The model under review builds one solid part; all positions refer to its coordinate system, in mm. A direction names the side the tool comes from. Round coordinates to 2 decimals unless told otherwise and drop trailing zeros. Order: outer loops, then holes, each group sorted by start corner. A loop starts at its lowest first (then second) coordinate and runs counter-clockwise, first axis right, second up. Notation, with made-up numbers: M 0.5,38.25 L 6.5,38.25 A16 ccw 6.5,62.25 Z; hole C 52,41.5 d8. An arc over 180 degrees is marked long. Use a Markdown table: item, result. Add a question column.
1. The part is to be moulded in two halves that separate along Y. For faces 1 (the cylindrical face through (43.544, 9.789, 10.874)), 2 (the cylindrical face through (-42.526, -11.023, -1.496)), 3 (the flat face through (44, 6.215, 16)), 4 (the flat face through (-41.952, -7, 10)), say which applies: +Y half, -Y half, draft (parallel to the pull), parting line (faces both ways), or undercut.
2. Consider section D-D on y = -10. State the section outline as (x, z) points, then the cut area to 3 significant figures.
3. Insertion check: P1, Ø0.6, axis at x = 44, y = 0.5, coming from the +Z side; P2, Ø0.6, axis at x = 44, z = 17, coming from the +Y side; P3, Ø2, axis at x = -43.5, z = 15, coming from the +Y side. Each pin has a flat end and moves straight along its axis. Give the tip position at first contact, or say it passes through.
4. Consider section C-C on x = 15.5. State the section outline as (y, z) points.
5. For faces 5 (the flat face through (44, 1, 10)), 6 (the flat face through (0, -11, 0)), 7 (the flat face through (-43, -17.785, 16)), list the 3-axis set-ups (+Z, -Z, +X, -X, +Y, -Y) from which the entire face can be reached by the end or side of a thin tool; tool diameter is ignored.
6. To check wall thickness, follow probe 1 along Y at (x, z) = (-22, 3.5); probe 2 along X at (y, z) = (-15, 11.5); probe 3 along Z at (x, y) = (4, -22). State the ranges of each line that lie inside material, in increasing order.
7. Consider section A-A on z = 15. State the section outline as (x, y) points.
8. Consider section B-B on z = 4.25. State the section outline as (x, y) points.
from build123d import *

# Parameters (mm, degrees)
F0_W      = 89
F0_H      = 44
F0_W_2    = 85
F0_H_2    = 40
F1_DEPTH  = 20
F2_W      = 89
F2_H      = 44
F2_W_2    = 85
F2_H_2    = 40
F3_DEPTH  = 3
F4_R      = 5
F5_R      = 3
F6_W      = 10
F6_H      = 10
F7_DEPTH  = 3
F8_W      = 10
F8_H      = 10
F9_DEPTH  = 3
F10_R     = 1.5
F12_DEPTH = 25


with BuildPart() as f1:
    # F0 (on Top) → F1 (new body)
    with BuildSketch(Plane.XY):
        with Locations((0.5476979613, -10.7853626366)):
            Rectangle(F0_W, F0_H)
        with Locations((0.5476979613, -10.7853626366)):
            Rectangle(F0_W_2, F0_H_2, mode=Mode.SUBTRACT)
    extrude(amount=F1_DEPTH)

    # F2 (on face) → F3 (join)
    with BuildSketch(Plane(origin=(0, 0, 0), x_dir=(1, 0, 0), z_dir=(0, 0, -1))):
        with Locations((0.5476979613, 10.7853626366)):
            Rectangle(F2_W, F2_H)
        with Locations((0.5476979613, 10.7853626366)):
            Rectangle(F2_W_2, F2_H_2, mode=Mode.SUBTRACT)
        with Locations((0.5476979613, 10.7853626366)):
            Rectangle(F2_W_2, F2_H_2)
    extrude(amount=F3_DEPTH)

    # F4
    f4_edges = [f1.edges().sort_by_distance(p)[0] for p in [
        (-43.952302, -32.785363, 8.5),
        (45.047698, -32.785363, 8.5),
        (45.047698, 11.214637, 8.5),
        (-43.952302, 11.214637, 8.5),
        (-43.952302, -10.785363, -3),
        (0.547698, 11.214637, -3),
        (45.047698, -10.785363, -3),
        (0.547698, -32.785363, -3),
    ]]
    fillet(f4_edges, radius=F4_R)

    # F5
    f5_edges = [f1.edges().sort_by_distance(p)[0] for p in [
        (-41.952302, 9.214637, 10),
        (-41.952302, -30.785363, 10),
        (43.047698, 9.214637, 10),
        (43.047698, -30.785363, 10),
    ]]
    fillet(f5_edges, radius=F5_R)

    # F6 (on face) → F7 (cut)
    with BuildSketch(Plane.YZ.offset(45.0476979613)):
        with Locations((1.2146373634, 15)):
            Rectangle(F6_W, F6_H)
    extrude(amount=-F7_DEPTH, mode=Mode.SUBTRACT)

    # F8 (on face) → F9 (cut)
    with BuildSketch(Plane(origin=(-43.9523020387, 0, 0), x_dir=(0, -1, 0), z_dir=(-1, 0, 0))):
        with Locations((22.7853626366, 15)):
            Rectangle(F8_W, F8_H)
    extrude(amount=-F9_DEPTH, mode=Mode.SUBTRACT)

    # F10
    f10_edges = [f1.edges().sort_by_distance(p)[0] for p in [
        (44.047698, 6.214637, 10),
        (44.047698, -3.785363, 10),
        (-42.952302, -27.785363, 10),
        (-42.952302, -17.785363, 10),
    ]]
    fillet(f10_edges, radius=F10_R)

    # F11 (on face) → F12 (cut)
    with BuildSketch(Plane(origin=(0, 0, -3), x_dir=(1, 0, 0), z_dir=(0, 0, -1))):
        with BuildLine():
            ThreePointArc((18.5476979613, 12.7853626366), (16.9367852579, 16.6744499331), (13.0476979613, 18.2853626366))
            ThreePointArc((13.0476979613, 18.2853626366), (9.1586106648, 8.89627534), (18.5476979613, 12.7853626366))
        make_face()
    extrude(amount=-F12_DEPTH, mode=Mode.SUBTRACT)


with BuildPart() as f13_1:
    # F13: copy of F1
    add(f1.part.moved(Location((0, 0, 30))))


solid = f1.part
Answer block:
| question | item | result |
|---|---|---|
| 1 | face 1 | +Y half |
| 1 | face 2 | draft |
| 1 | face 3 | undercut |
| 1 | face 4 | undercut |
| 2 | outline | M -43.95,2 A5 ccw -38.95,-3 L 8.31,-3 L 8.31,0 L -41.95,0 L -41.95,20 L -43.95,20 Z; M 17.79,-3 L 40.05,-3 A5 ccw 45.05,2 L 45.05,20 L 43.05,20 L 43.05,0 L 17.79,0 Z |
| 2 | area | 308 mm^2 |
| 3 | P1 | z = 10 |
| 3 | P2 | y = 9.63 |
| 3 | P3 | y = 9.74 |
| 4 | outline | M -32.79,2 A5 ccw -27.79,-3 L -17.71,-3 L -17.71,0 L -30.79,0 L -30.79,20 L -32.79,20 Z; M -7.86,-3 L 6.21,-3 A5 ccw 11.21,2 L 11.21,20 L 9.21,20 L 9.21,0 L -7.86,0 Z |
| 5 | face 5 | +Z, +X |
| 5 | face 6 | +Z |
| 5 | face 7 | +Z, -X |
| 6 | probe 1 | -32.79 to -30.79, 9.21 to 11.21 |
| 6 | probe 2 | -43.95 to -41.95, 43.05 to 45.05 |
| 6 | probe 3 | -3 to 0 |
| 7 | outline | M -43.95,-27.79 A5 ccw -38.95,-32.79 L 40.05,-32.79 A5 ccw 45.05,-27.79 L 45.05,-3.79 L 43.05,-3.79 L 43.05,-27.79 A3 cw 40.05,-30.79 L -38.95,-30.79 A3 cw -41.95,-27.79 Z; M -43.95,-17.79 L -41.95,-17.79 L -41.95,6.21 A3 cw -38.95,9.21 L 40.05,9.21 A3 cw 43.05,6.21 L 45.05,6.21 A5 ccw 40.05,11.21 L -38.95,11.21 A5 ccw -43.95,6.21 Z |
| 8 | outline | M -43.95,-27.79 A5 ccw -38.95,-32.79 L 40.05,-32.79 A5 ccw 45.05,-27.79 L 45.05,6.21 A5 ccw 40.05,11.21 L -38.95,11.21 A5 ccw -43.95,6.21 Z; hole M -41.95,-27.79 A3 ccw -38.95,-30.79 L 40.05,-30.79 A3 ccw 43.05,-27.79 L 43.05,6.21 A3 ccw 40.05,9.21 L -38.95,9.21 A3 ccw -41.95,6.21 Z |
